Can you work these out from the model? Positions are in its coordinate system, mm. A direction names the side the tool comes from. Round coordinates to 2 decimals unless told otherwise and drop trailing zeros. Loops run counter-clockwise (first coordinate to the right, second up) from the corner with the lowest first, then second, coordinate; pieces in that order, holes last. Notation, with made-up numbers: (42, 54.25) - (53, 54.25) arc R14 ccw to (53, 78.25) - close; hole circle Ø9 at (-30.5, -33.75). An arc over 180 degrees is marked (long way). Answer as CSV lines item,"result".
```python
from build123d import *

# Parameters (mm, degrees)
SM_BASE_FLANGE_1_DEPTH = 48
CUT_EXTRUDE_1_DEPTH    = 10
SKETCH_10_R            = 3.5
CUT_EXTRUDE_2_DEPTH    = 10
SKETCH_11_W            = 30
SKETCH_11_H            = 26
CUT_EXTRUDE_3_DEPTH    = 15
OTHER_START            = 16.263455967
OTHER_1_OUTLINE_W      = 4
OTHER_1_OUTLINE_H      = 30.405591591
OTHER_1_DEPTH          = 3.535533906
OTHER_START_2          = 59.75052301
OTHER_1_2_OUTLINE_W    = 4
OTHER_1_2_OUTLINE_H    = 30.405591591
OTHER_1_2_DEPTH        = 3.535533906
OTHER_START_3          = 30.405591591
OTHER_1_3_OUTLINE_W    = 4
OTHER_1_3_OUTLINE_H    = 3.594408409
OTHER_1_3_DEPTH        = 7.071067812


# Read off the part's stored shape, not the designer's step: Затупленный угол1
# Sheet-metal steps are written as plain solids
with BuildPart() as part:
    # Sketch 2 → Базовая кромка1 (new body)
    with BuildSketch(Plane.XY):
        with BuildLine():
            Line((0, 0), (0, 53.5))
            ThreePointArc((0, 53.5), (0.878679656, 55.621320344), (3, 56.5))
            Line((3, 56.5), (22, 56.5))
            ThreePointArc((22, 56.5), (24.121320344, 55.621320344), (25, 53.5))
            Line((25, 53.5), (25, 46.5))
            Line((25, 46.5), (23.5, 46.5))
            Line((23.5, 46.5), (23.5, 53.5))
            ThreePointArc((23.5, 53.5), (23.060660172, 54.560660172), (22, 55))
            Line((22, 55), (3, 55))
            ThreePointArc((3, 55), (1.939339828, 54.560660172), (1.5, 53.5))
            Line((1.5, 53.5), (1.5, 0))
            Line((1.5, 0), (0, 0))
        make_face()
    extrude(amount=SM_BASE_FLANGE_1_DEPTH)

    # Эскиз7 → Вырез-Вытянуть1 (cut)
    with BuildSketch(Plane.ZY):
        Polygon((23, 0), (23, 26.720943809), (0, 40), (0, 0), align=None)
    extrude(amount=-CUT_EXTRUDE_1_DEPTH, mode=Mode.SUBTRACT)

    # Эскиз10 → Вырез-Вытянуть2 (cut)
    with BuildSketch(Plane.ZY):
        with Locations((38, 10)):
            Circle(SKETCH_10_R)
        with Locations((38, 30)):
            Circle(SKETCH_10_R)
    extrude(amount=-CUT_EXTRUDE_2_DEPTH, mode=Mode.SUBTRACT)

    # Эскиз11 → Вырез-Вытянуть3 (cut)
    with BuildSketch(Plane(origin=(0, 56.5, 0), x_dir=(1, 0, 0), z_dir=(0, 1, 0))):
        with Locations((11, -35)):
            Rectangle(SKETCH_11_W, SKETCH_11_H)
    extrude(amount=-CUT_EXTRUDE_3_DEPTH, mode=Mode.SUBTRACT)

    # Other 1 outline → Other 1 (cut)
    with BuildSketch(Plane(origin=(0, 0, 0), x_dir=(1, 0, 0), z_dir=(0, 0.707106781186547, 0.707106781186548)).offset(OTHER_START)):
        with Locations((1, -15.202795796)):
            Rectangle(OTHER_1_OUTLINE_W, OTHER_1_OUTLINE_H)
    extrude(amount=OTHER_1_DEPTH, mode=Mode.SUBTRACT)

    # Other 1 2 outline → Other 1 2 (cut)
    with BuildSketch(Plane(origin=(0, 0, 0), x_dir=(1, 0, 0), z_dir=(0, 0.707106781186547, 0.707106781186548)).offset(OTHER_START_2)):
        with Locations((1, -15.202795796)):
            Rectangle(OTHER_1_2_OUTLINE_W, OTHER_1_2_OUTLINE_H)
    extrude(amount=OTHER_1_2_DEPTH, mode=Mode.SUBTRACT)

    # Other 1 3 outline → Other 1 3 (cut)
    with BuildSketch(Plane(origin=(0, 0, 0), x_dir=(1, 0, 0), z_dir=(0, 0.707106781186547, 0.707106781186548)).offset(OTHER_START_3)):
        with Locations((1, -32.202795796)):
            Rectangle(OTHER_1_3_OUTLINE_W, OTHER_1_3_OUTLINE_H)
    extrude(amount=OTHER_1_3_DEPTH, mode=Mode.SUBTRACT)


solid = part.part
```
Q1. Imagine slicing it at D-D (z = 19.5). Write out the boundary of the cut face in (x, y).
Checks:
outline,"(0, 28.74) - (1.5, 28.74) - (1.5, 53.5) arc R1.5 cw to (3, 55) - (22, 55) arc R1.5 cw to (23.5, 53.5) - (23.5, 46.5) - (25, 46.5) - (25, 53.5) arc R3 ccw to (22, 56.5) - (3, 56.5) arc R3 ccw to (0, 53.5) - close"
Q2. Imagine slicing it at C-C (x = 4). Write out the boundary of the cut face in (y, z), then the cut area to 3 significant figures.
Checks:
outline,"(55, 0) - (56.5, 0) - (56.5, 22) - (55, 22) - close"
area,"33.0 mm²"
Q3. If I drill on line 1 along Y through (x, z) = (0.95, 38); line 2 along X through (y, z) = (17, 31.5); line 3 along Y through (x, z) = (1, 33), over which ranges is the centre line in solid material (lowest first)? Write a range as [from, to].
Checks:
line 1,"[0, 6.5], [13.5, 26.5], [33.5, 41.5]"
line 2,"[0, 1.5]"
line 3,"[0, 41.5]"
Q4. Imagine slicing it at A-A (y = 10). Write out the boundary of the cut face in (x, z), then the cut area to 3 significant figures.
Checks:
outline,"(0, 23) - (1.5, 23) - (1.5, 34.5) - (0, 34.5) - close; (0, 41.5) - (1.5, 41.5) - (1.5, 48) - (0, 48) - close"
area,"27.0 mm²"
Q5. On a 3-axis mill with a long thin cutter (end or side, diameter ignored), from which of +Z, -Z, +X, -X, +Y, -Y can I reach the whole of each face in a straight line? I mean faces 4 (the flat face through (10, 56, 0)), 5 (the flat face through (1, 41.5, 32)), 6 (the flat face through (13, 55, 11)), 7 (the cylindrical face through (0.7, 7.9, 35.2)), 8 (the flat face through (1, 16, 23)). Say none if no direction works.
Checks:
face 4,"-Z, +X, -X, +Y, -Y"
face 5,"+Z, +X, -X, +Y"
face 6,"+Z, -Z, -Y"
face 7,"+X, -X"
face 8,"-Z, +X, -X, -Y"
Q6. Imagine slicing it at B-B (z = 38). Write out the boundary of the cut face in (x, y).
Checks:
outline,"(0, 0) - (1.5, 0) - (1.5, 6.5) - (0, 6.5) - close; (0, 13.5) - (1.5, 13.5) - (1.5, 26.5) - (0, 26.5) - close; (0, 33.5) - (1.5, 33.5) - (1.5, 41.5) - (0, 41.5) - close"
Q7. We'd pull the mould along X, two halves only. Please class faces 1 (the cylindrical face through (24.1, 55.64, 10.85)), 2 (the flat face through (12, 56.5, 11)), 3 (the flat face through (23.5, 50, 11)): pulls with the +X half, pulls with the -X half, needs draft (parallel to the pull), parting line crosses it, or undercut.
Checks:
face 1,"pulls with the +X half"
face 2,"needs draft"
face 3,"undercut"
Q8. I'm going to push flat-ended pins straight in: pin 1 Ø9.5 at (x, z) = (16, 10) entering from -Y; pin 2 Ø5 at (y, z) = (39.5, 26) entering from +X; pin 3 Ø1.6 at (x, z) = (0.5, 27.5) entering from +Y. Where does each tip first touch, or does it pass through?
Checks:
pin 1,"y = 55"
pin 2,"x = 1.5"
pin 3,"y = 41.5"
